Source: CAD feature listing. Evaluate the final solid. Frame: model axes, mm. A direction names the side the tool comes from. Round coordinates to 2 decimals unless told otherwise and drop trailing zeros. Order: outer loops, then holes, each group sorted by start corner. A loop starts at its lowest first (then second) coordinate and runs counter-clockwise, first axis right, second up. Notation, with made-up numbers: (-2, 78) -> (32, 78) arc R17 ccw to (32, 107) -> close; hole circle Ø8 at (48, 58). An arc over 180 degrees is marked (long way). Answer as CSV lines item,"result". Start each with the question number.
(1) Contact query for flat-ended pins moving along their axis: P1, Ø0.7, axis at x = -1.5, y = 0.5, coming from the -Z side; P2, Ø9, axis at x = -3.5, z = 56, coming from the +Y side; P3, Ø1.2, axis at y = 0, z = 53, coming from the +X side; P4, Ø5, axis at x = 4.5, y = -2, coming from the -Z side. Output: stop coordinate, or through.
(2) Section query C-C (x = 24.5). Output: boundary loops of the cut face in (y, z), plus the area to 3 significant figures.
(3) Section query D-D (x = 113.5). Output: boundary loops of the cut face in (y, z).
(4) Pull-direction query (Z, two-part tool) for faces 6 (the flat face through (37.3, 0, 58)), 7 (the flat face through (23, 0, 90)), 8 (the flat face through (-5, 1.2, 5)); classes: +Z half, -Z half, draft (parallel to the pull), parting line (faces both ways), or undercut.
(5) Line query: line 1 along X through (y, z) = (5.25, 92.5); line 2 along X through (y, z) = (-4, 94); line 3 along X through (y, z) = (1, 13). Output: solid intervals per line, ascending. Write a range as from..to.
(6) Section query B-B (z = 65.5). Output: boundary loops of the cut face in (x, y).
(7) Set-up query: faces 1 (the flat face through (60, 12, 64)), 2 (the flat face through (-5, 1.2, 56)), 3 (the flat face through (14, 0, 50)), 4 (the flat face through (167.1, 0, 97)), 5 (the cylindrical face through (48.71, 0.17, 97.87)). Return all of +Z, -Z, +X, -X, +Y, -Y with unobstructed straight access to the full face (end or side cutting, diameter ignored); none if empty.
(8) Section query A-A (y = -7.75). Output: boundary loops of the cut face in (x, z).
Autodesk Fusion 360 part; units mm, degrees
sketch "Arm triangle" plane through (0, 0, 0) normal (0, 1, 0) x (1, 0, 0)
  line L0 (0, 0) -> (0, -90)
  line L1 (0, -90) -> (150, -90)
  line L2 (150, -90) -> (0, 0)
  dimension "d186" = 90
extrude "Arm triangle (1)" add sketch "Arm triangle" along normal mid plane 24
sketch "Plate" plane through (0, 0, 0) normal (0, 1, 0) x (1, 0, 0)
  line L0 (0, 0) -> (6, 0)
  line L1 (6, 0) -> (6, -90)
  line L2 (6, -90) -> (0, -90)
  line L3 (0, -90) -> (0, 0)
  dimension "d190" = 6
  dimension "d191" = 90
extrude "Plate (1)" add sketch "Plate" along normal mid plane 24
sketch "Lightening cutout" plane through (0, 0, 0) normal (0, 1, 0) x (1, 0, 0)
  line L0 (14, -24.7267) -> (14, -76)
  line L1 (14, -76) -> (37.3, -76)
  line L2 (37.3, -76) -> (37.3, -38.7067)
  line L3 (37.3, -38.7067) -> (14, -24.7267)
  dimension "d194" = 14
  dimension "d195" = 24.7267
  dimension "d196" = 76
  dimension "d197" = 37.3
  dimension "d198" = 38.7067
extrude "Lightening cutout (1)" cut sketch "Lightening cutout" along normal mid plane 34
sketch "Saddle boss x=70" plane through (0, 0, 0) normal (0, 1, 0) x (1, 0, 0)
  circle A0 centre (70, -90) radius 22.7
  dimension "d201" = 70
  dimension "d202" = 90
  dimension "d203" = 45.4
extrude "Saddle boss x=70 (1)" add sketch "Saddle boss x=70" along normal mid plane 24
sketch "Saddle boss x=150" plane through (0, 0, 0) normal (0, 1, 0) x (1, 0, 0)
  circle A0 centre (150, -90) radius 22.7
  dimension "d207" = 90
  dimension "d208" = 45.4
extrude "Saddle boss x=150 (1)" add sketch "Saddle boss x=150" along normal mid plane 24
sketch "Rod pocket x=70" plane through (0, 0, 0) normal (0, 1, 0) x (1, 0, 0)
  circle A0 centre (70, -90) radius 17.1
  dimension "d211" = 70
  dimension "d212" = 90
  dimension "d213" = 34.2
extrude "Rod pocket x=70 (1)" cut sketch "Rod pocket x=70" along normal mid plane 34
sketch "Drop-in opening x=70" plane through (0, 0, 0) normal (0, 1, 0) x (1, 0, 0)
  line L0 (52.9, -90) -> (87.1, -90)
  line L1 (87.1, -90) -> (87.1, -117.7)
  line L2 (87.1, -117.7) -> (52.9, -117.7)
  line L3 (52.9, -117.7) -> (52.9, -90)
  dimension "d216" = 52.9
  dimension "d217" = 90
  dimension "d218" = 87.1
  dimension "d219" = 117.7
extrude "Drop-in opening x=70 (1)" cut sketch "Drop-in opening x=70" along normal mid plane 34
sketch "Rod pocket x=150" plane through (0, 0, 0) normal (0, 1, 0) x (1, 0, 0)
  circle A0 centre (150, -90) radius 17.1
  dimension "d223" = 90
  dimension "d224" = 34.2
extrude "Rod pocket x=150 (1)" cut sketch "Rod pocket x=150" along normal mid plane 34
sketch "Drop-in opening x=150" plane through (0, 0, 0) normal (0, 1, 0) x (1, 0, 0)
  line L0 (132.9, -90) -> (167.1, -90)
  line L1 (167.1, -90) -> (167.1, -117.7)
  line L2 (167.1, -117.7) -> (132.9, -117.7)
  line L3 (132.9, -117.7) -> (132.9, -90)
  dimension "d227" = 132.9
  dimension "d228" = 90
  dimension "d229" = 167.1
  dimension "d230" = 117.7
extrude "Drop-in opening x=150 (1)" cut sketch "Drop-in opening x=150" along normal mid plane 34
sketch "Hook profile" plane through (0, 0, 0) normal (0, 1, 0) x (1, 0, 0)
  line L0 (0, -88) -> (-8.3, -88)
  line L1 (-8.3, -88) -> (-8.3, -71)
  line L2 (-8.3, -71) -> (-5.3, -71)
  line L3 (-5.3, -71) -> (-3.8, -72.5)
  line L4 (-3.8, -72.5) -> (-3.8, -83)
  line L5 (-3.8, -83) -> (0, -83)
  line L6 (0, -83) -> (0, -88)
  dimension "d233" = 88
  dimension "d234" = 8.3
  dimension "d235" = 3.8
  dimension "d236" = 5
  dimension "d237" = 10.5
  dimension "d238" = 1.5
  dimension "d239" = 1.5
extrude "Hook profile (1)" add sketch "Hook profile" along normal mid plane 2.4
pattern_linear "Hook rows" count 4 spacing 25.4 along (0, 0, -1) count 3 spacing 0 along (0, 0, 1) of "Hook profile (1)"
equation "bracketWidth = 24.0 mm"
equation "hookTabWidth = slotWidth - 0.8 mm"
equation "slotPitchVertical = 25.4 mm"
equation "slotWidth = 3.2 mm"
equation "faceMetalThickness = 2.0 mm"
equation "hookThroat = faceMetalThickness + 1.8 mm"
equation "hookNeckHeight = 5.0 mm"
equation "hookLipThickness = 4.5 mm"
equation "hookLipDrop = 12.0 mm"
equation "plateThickness = 6.0 mm"
equation "plateHeight = 90.0 mm"
equation "rodOuterDiameter = 33.4 mm"
equation "saddleClearance = 0.8 mm"
equation "saddleWall = 6.0 mm"
equation "rearRodStandoff = 70.0 mm"
equation "rodSpacing = 80.0 mm"
equation "memberWidth = 14.0 mm"
equation "hookLipChamfer = 1.5 mm"
equation "topHookNeckTop = 88.0 mm"
equation "d186 = plateHeight"
equation "d188 = bracketWidth"
equation "d190 = plateThickness"
equation "d191 = plateHeight"
equation "d192 = bracketWidth"
equation "d194 = memberWidth"
equation "d195 = Linear Dimension-3"
equation "d196 = plateHeight - memberWidth"
equation "d197 = rearRodStandoff - ( rodOuterDiameter + 2 * saddleWall ) / 2 - 10 mm"
equation "d198 = Linear Dimension-6"
equation "d199 = bracketWidth + 10 mm"
equation "d201 = rearRodStandoff"
equation "d202 = plateHeight"
equation "d203 = rodOuterDiameter + 2 * saddleWall"
equation "d204 = bracketWidth"
equation "d207 = plateHeight"
equation "d208 = rodOuterDiameter + 2 * saddleWall"
equation "d209 = bracketWidth"
equation "d211 = rearRodStandoff"
equation "d212 = plateHeight"
equation "d213 = rodOuterDiameter + saddleClearance"
equation "d214 = bracketWidth + 10 mm"
equation "d216 = rearRodStandoff - ( rodOuterDiameter + saddleClearance ) / 2"
equation "d217 = plateHeight"
equation "d218 = rearRodStandoff + ( rodOuterDiameter + saddleClearance ) / 2"
equation "d219 = plateHeight + ( rodOuterDiameter + 2 * saddleWall ) / 2 + 5 mm"
equation "d220 = bracketWidth + 10 mm"
equation "d223 = plateHeight"
equation "d224 = rodOuterDiameter + saddleClearance"
equation "d225 = bracketWidth + 10 mm"
equation "d227 = ( rearRodStandoff + rodSpacing ) - ( rodOuterDiameter + saddleClearance ) / 2"
equation "d228 = plateHeight"
equation "d229 = ( rearRodStandoff + rodSpacing ) + ( rodOuterDiameter + saddleClearance ) / 2"
equation "d230 = plateHeight + ( rodOuterDiameter + 2 * saddleWall ) / 2 + 5 mm"
equation "d231 = bracketWidth + 10 mm"
equation "d233 = topHookNeckTop"
equation "d234 = hookThroat + hookLipThickness"
equation "d235 = hookThroat"
equation "d236 = hookNeckHeight"
equation "d237 = hookLipDrop - hookLipChamfer"
equation "d238 = hookLipChamfer"
equation "d239 = hookLipChamfer"
equation "d240 = hookTabWidth"
Answer block:
1,P1,"z = 6.8"
1,P2,"y = 12"
1,P3,"x = 89.33"
1,P4,"z = 0"
2,outline,"(-12, 14.7) -> (12, 14.7) -> (12, 31.03) -> (-12, 31.03) -> close; (-12, 76) -> (12, 76) -> (12, 90) -> (-12, 90) -> close"
2,area,"728 mm2"
3,outline,"(-12, 68.1) -> (12, 68.1) -> (12, 90) -> (-12, 90) -> close"
4,face 6,"undercut"
4,face 7,"+Z half"
4,face 8,"draft"
5,line 1,"47.44..52.9, 87.1..92.56, 127.44..132.9, 167.1..172.56"
5,line 2,"47.66..52.9, 87.1..92.34, 127.66..132.9, 167.1..172.34"
5,line 3,"0..21.67"
6,outline,"(0, -12) -> (14, -12) -> (14, 12) -> (0, 12) -> close; (37.3, -12) -> (109.17, -12) -> (109.17, 12) -> (37.3, 12) -> close"
7,face 1,"+Z, -Z, +X, -X, +Y"
7,face 2,"+Z, -Z, -X, +Y"
7,face 3,"+Y, -Y"
7,face 4,"+Z, +Y, -Y"
7,face 5,"+Z, -X, +Y, -Y"
8,outline,"(0, 0) -> (6, 0) -> (6, 3.6) -> (130.53, 78.32) arc R22.7 ccw (long way) to (167.1, 104.93) -> (167.1, 90) arc R17.1 cw to (132.9, 90) -> (132.9, 104.93) arc R22.7 ccw to (127.3, 90) -> (92.7, 90) arc R22.7 ccw to (87.1, 104.93) -> (87.1, 90) arc R17.1 cw to (52.9, 90) -> (52.9, 104.93) arc R22.7 ccw to (47.3, 90) -> (0, 90) -> close; hole (14, 24.73) -> (37.3, 38.71) -> (37.3, 76) -> (14, 76) -> close"
